Build history of the part. All positions in model axes, mm. A direction names the side the tool comes from. Coordinates: 2 decimals unless noted, no trailing zeros. Order: outer loops, then holes, each group sorted by start corner. A loop starts at its lowest first (then second) coordinate and runs counter-clockwise, first axis right, second up. Notation, with made-up numbers: (-22, 3.5) - (31, 3.5) arc R17 ccw to (31, 14.5) - close; hole circle Ø1 at (78.5, 64.25). An arc over 180 degrees is marked (long way). One line per item, written item: value.
from build123d import *

# Parameters (mm, degrees)
CROQUIS1_W              = 140
CROQUIS1_H              = 90
SALIENTE_EXTRUIR1_DEPTH = 10
CROQUIS2_W              = 140
CROQUIS2_H              = 10
SALIENTE_EXTRUIR2_DEPTH = 100
REDONDEO1_R             = 70
CORTAR_EXTRUIR1_DEPTH   = 100


with BuildPart() as part:
    # Croquis1 → Saliente-Extruir1 (new body)
    with BuildSketch(Plane(origin=(0, 0, 0), x_dir=(1, 0, 0), z_dir=(0, 1, 0))):
        Rectangle(CROQUIS1_W, CROQUIS1_H)
    extrude(amount=SALIENTE_EXTRUIR1_DEPTH)

    # Croquis2 → Saliente-Extruir2 (add)
    with BuildSketch(Plane(origin=(0, 10, 0), x_dir=(1, 0, 0), z_dir=(0, 1, 0))):
        with Locations((0, -40)):
            Rectangle(CROQUIS2_W, CROQUIS2_H)
        with Locations((0, 40)):
            Rectangle(CROQUIS2_W, CROQUIS2_H)
    extrude(amount=SALIENTE_EXTRUIR2_DEPTH)

    # Redondeo1
    redondeo1_edges = [part.edges().sort_by_distance(p)[0] for p in [
        (-70, 110, 40),
        (70, 110, 40),
        (70, 110, -40),
        (-70, 110, -40),
    ]]
    fillet(redondeo1_edges, radius=REDONDEO1_R - 0.0001)  # a hair under: the kernel refuses the full size

    # Croquis3 → Cortar-Extruir1 (cut)
    with BuildSketch(Plane.XY.offset(45)):
        with BuildLine():
            ThreePointArc((0, 93), (-20, 73), (0, 53))
            Line((0, 53), (0, 73))
            Line((0, 73), (0, 93))
        make_face()
        with BuildLine():
            Line((0, 73), (0, 53))
            ThreePointArc((0, 53), (14.142135624, 58.857864376), (20, 73))
            ThreePointArc((20, 73), (14.142135624, 87.142135624), (0, 93))
            Line((0, 93), (0, 73))
        make_face()
    extrude(amount=-CORTAR_EXTRUIR1_DEPTH, mode=Mode.SUBTRACT)


solid = part.part
1. 3-axis set-ups, long thin cutter, end or side, ignore diameter. For faces 4 (the face through (-1, 10, 0)), 5 (the face through (50.04, 88.95, -40.07)): which of +Z, -Z, +X, -X, +Y, -Y reach the whole face in a straight line?
Values found:
face 4: +X, -X, +Y
face 5: +Z, -Z, +X, +Y
2. Probe line 1 along Z through (x, y) = (-22.5, 103.5); line 2 along Y through (x, z) = (-49, -14); line 3 along Y through (x, z) = (9, 37). List the from-to ranges inside material, lowest first.
Values found:
line 1: z = -45 to -35, 35 to 45
line 2: y = 0 to 10
line 3: y = 0 to 55.14, 90.86 to 109.42
3. Band-saw the part on B-B, the plane x = 16.5. Give the cut face in (y, z).
Values found:
outline: (0, -45) - (61.7, -45) - (61.7, -35) - (10, -35) - (10, 35) - (61.7, 35) - (61.7, 45) - (0, 45) - close; (84.3, -45) - (108.03, -45) - (108.03, -35) - (84.3, -35) - close; (84.3, 35) - (108.03, 35) - (108.03, 45) - (84.3, 45) - close
4. Flat gauge pins, fed straight in: P1, Ø6, axis at x = -9.5, z = -6.5, coming from the -Y side; P2, Ø21, axis at x = 14, z = 14, coming from the +Y side. Where does each tip first touch, or does it go through?
Values found:
P1: stops at y = 0
P2: stops at y = 10
5. Band-saw the part on A-A, the plane y = 19.5. Give the cut face in (x, z), and give its area (3 significant figures).
Values found:
outline: (-70, -45) - (70, -45) - (70, -35) - (-70, -35) - close; (-70, 35) - (70, 35) - (70, 45) - (-70, 45) - close
area: 2,800 mm2
6. Band-saw the part on D-D, the plane x = -38.5. Give the cut face in (y, z).
Values found:
outline: (0, -45) - (98.46, -45) - (98.46, -35) - (10, -35) - (10, 35) - (98.46, 35) - (98.46, 45) - (0, 45) - close
7. Band-saw the part on C-C, the plane y = 66. Give the cut face in (x, z) (3 decimals).
Values found:
outline: (-64.992, -45) - (-18.735, -45) - (-18.735, -35) - (-64.992, -35) - close; (-64.992, 35) - (-18.735, 35) - (-18.735, 45) - (-64.992, 45) - close; (18.735, -45) - (64.992, -45) - (64.992, -35) - (18.735, -35) - close; (18.735, 35) - (64.992, 35) - (64.992, 45) - (18.735, 45) - close
8. Two-plate mould, pull along Z, no slides. Class faces 1 (the face through (-1, 42, -45)), 2 (the face through (-50.04, 88.95, -40.07)), 3 (the face through (-1, 48, 35)): pulls with the +Z half, pulls with the -Z half, needs draft (parallel to the pull), parting line crosses it, or undercut.
Values found:
face 1: pulls with the -Z half
face 2: needs draft
face 3: undercut
